Verification items for the finished model (mm, model axes). A direction names the side the tool comes from. Give positions to 0.01 mm unless a question says otherwise; leave off trailing zeros. Write each loop counter-clockwise with the first axis right and the second up, starting at its lowest first coordinate (ties: lowest second). Pieces come first, ordered by that corner, then holes. Notation, with made-up numbers: (14, 75) - (26, 75) arc R15 ccw to (26, 87) - close; hole circle Ø5 at (42, 15.25). An arc over 180 degrees is marked (long way). Answer as a JSON object with one key per item and string values. Group by question number.
Item 1: Go/stop test with flat-tipped pins: pin 1 (2 mm diameter, centred on x = -34.5, y = -88, fed in from -Z); pin 2 (14 mm diameter, centred on y = -80, z = 18, fed in from +X); pin 3 (1 mm diameter, centred on x = 27, y = -97, fed in from +Z). Record where each tip stops, or that it passes through.
Item 2: Sectioned sample at A-A, the plane x = -23. Record the boundary of the cut face in (y, z), and give its area (3 significant figures).
Item 3: Scan lines: line 1 along X through (y, z) = (-75.5, 29.5); line 2 along X through (y, z) = (-106, 2.5); line 3 along Z through (x, y) = (-38.5, -106). Record each from-to range of solid material in increasing order. Write a range as [from, to].
Item 4: Sectioned sample at B-B, the plane y = -99. Record the boundary of the cut face in (x, z).
Item 5: Tool access check on faces 1 (the face through (-0.602, -67.05, 30.875)), 2 (the face through (29.8, -88.5, 19)), 3 (the face through (-4.43, -106.75, 7.51)), 4 (the face through (43.99, -93.07, 12.73)). Record the directions out of +Z, -Z, +X, -X, +Y, -Y that give a thin tool (end or side, any length) a straight path to the whole face; none if there is none.
Item 6: Draft check along Y on faces 5 (the face through (-4.427, -71.074, 32.395)), 6 (the face through (-43, -100, 8)), 7 (the face through (-36.021, -104.645, 6.237)). Enter one of: +Y half, -Y half, draft (parallel to the pull), parting line (faces both ways), or undercut.
Item 7: Sectioned sample at C-C, the plane z = 17. Record the boundary of the cut face in (x, y).
Item 8: Sectioned sample at D-D, the plane x = -35.5. Record the boundary of the cut face in (y, z), and give its area (3 significant figures).
```python
from build123d import *

# Parameters (mm, degrees)
SKETCH019_W             = 90
SKETCH019_H             = 52.43
PAD008_DEPTH            = 7
SKETCH020_W             = 86
SKETCH020_H             = 48.43
POCKET010_DEPTH         = 5
SKETCH030_W             = 67
SKETCH030_H             = 41.5
PAD011_DEPTH            = 2.5
SKETCH021_W             = 61
SKETCH021_H             = 43.5
POCKET011_DEPTH         = 7.001
SKETCH029_W             = 90
SKETCH029_H             = 15
POCKET016_DEPTH         = 5
BODY001_PLACEMENT_ANGLE = 34.9


with BuildPart() as part:
    # Sketch019 → Pad008 (new body)
    with BuildSketch(Plane.XY):
        with Locations((0, 26.215)):
            Rectangle(SKETCH019_W, SKETCH019_H)
    extrude(amount=PAD008_DEPTH)

    # Sketch020 (on Face5 of Pad008) → Pocket010 (cut)
    with BuildSketch(Plane(origin=(0, 0, 0), x_dir=(1, 0, 0), z_dir=(0, 0, -1))):
        with Locations((0, -26.215)):
            Rectangle(SKETCH020_W, SKETCH020_H)
    extrude(amount=-POCKET010_DEPTH, mode=Mode.SUBTRACT)

    # Sketch030 (on Face11 of Pocket010) → Pad011 (join)
    with BuildSketch(Plane(origin=(0, 0, 5), x_dir=(1, 0, 0), z_dir=(0, 0, -1))):
        with Locations((-4, -26.25)):
            Rectangle(SKETCH030_W, SKETCH030_H)
    extrude(amount=PAD011_DEPTH)

    # Sketch021 (on Face5 of Pocket010) → Pocket011 (cut, through all)
    with BuildSketch(Plane.XY.offset(7)):
        with Locations((-4, 26.25)):
            Rectangle(SKETCH021_W, SKETCH021_H)
    extrude(amount=-POCKET011_DEPTH, mode=Mode.SUBTRACT)

    # Sketch029 (on Face4 of Pocket011) → Pocket016 (cut)
    with BuildSketch(Plane(origin=(0, 0, 0), x_dir=(1, 0, 0), z_dir=(0, 0, -1))):
        with Locations((0, -26.21)):
            Rectangle(SKETCH029_W, SKETCH029_H)
    extrude(amount=-POCKET016_DEPTH, mode=Mode.SUBTRACT)


with BuildPart() as part_1:
    # Body001 placement: moved
    add(part.part.moved(Location((0, -107, 0))).rotate(Axis((0, -107, 0), (1, 0, 0)), BODY001_PLACEMENT_ANGLE))


solid = part_1.part
```
Geometry check:
{
 "1": {"pin 1": "z = 18.65", "pin 2": "x = 45", "pin 3": "z = 15.86"},
 "2": {"outline": "(-111.01, 5.74) - (-107, 0) - (-105.36, 1.14) - (-108.22, 5.25) - (-106.17, 6.68) - (-107.31, 8.32) - close; (-71.64, 33.2) - (-70.49, 31.56) - (-68.5, 32.95) - (-65.64, 28.85) - (-64, 30) - (-68, 35.74) - close", "area": "37.9 mm^2"},
 "3": {"line 1": "[-45, -34.5], [26.5, 45]", "line 2": "[-45, -43], [43, 45]", "line 3": "[0.7, 2.06], [6.79, 9.23]"},
 "4": {"outline": "(-45, 5.58) - (-43, 5.58) - (-43, 11.68) - (-37.5, 11.68) - (-37.5, 8.63) - (-34.5, 8.63) - (-34.5, 14.12) - (-45, 14.12) - close; (26.5, 8.63) - (29.5, 8.63) - (29.5, 11.68) - (43, 11.68) - (43, 5.58) - (45, 5.58) - (45, 14.12) - (26.5, 14.12) - close"},
 "5": {"face 1": "-Z", "face 2": "none", "face 3": "+Z, +Y", "face 4": "+X, -X, +Y"},
 "6": {"face 5": "-Y half", "face 6": "draft", "face 7": "undercut"},
 "7": {"outline": "(-45, -94.87) - (-34.5, -94.87) - (-34.5, -91.37) - (-45, -91.37) - close; (26.5, -94.87) - (45, -94.87) - (45, -91.37) - (26.5, -91.37) - close"},
 "8": {"outline": "(-111.01, 5.74) - (-107, 0) - (-105.36, 1.14) - (-108.22, 5.25) - (-105.35, 7.25) - (-103.92, 5.2) - (-93.09, 12.76) - (-94.52, 14.81) - (-82.21, 23.39) - (-80.78, 21.34) - (-69.88, 28.94) - (-71.31, 30.99) - (-68.5, 32.95) - (-65.64, 28.85) - (-64, 30) - (-68, 35.74) - close", "area": "191 mm^2"}
}
